Part model, mm, in its own coordinate system. Coordinates: 2 decimals unless noted, no trailing zeros. Write each loop counter-clockwise with the first axis right and the second up, starting at its lowest first coordinate (ties: lowest second). Pieces come first, ordered by that corner, then holes. Notation, with made-up numbers: (-25, 53.5) - (-17, 53.5) arc R5 ccw to (-17, 61.5) - close; hole circle Ø8 at (-27, 67). An arc over 180 degrees is marked (long way). Use a Markdown table: item, result.
```python
from build123d import *

# Parameters (mm, degrees)
SKETCH2_W           = 630
SKETCH2_H           = 6.2
SKETCH2_W_2         = 51.63
SKETCH2_H_2         = 51.63
BOSS_EXTRUDE1_DEPTH = 30
SKETCH2_5_W         = 14
SKETCH2_5_H         = 99
BOSS_EXTRUDE2_DEPTH = 14


with BuildPart() as part:
    # Sketch2 → Boss-Extrude1 (new body)
    # profile 1 of 2: a face of its own
    with BuildSketch(Plane(origin=(0, 0, 0), x_dir=(1, 0, 0), z_dir=(0, 1, 0))):
        Polygon((-320, -34), (-320, -65), (320, -65), (320, -34), (320, 65), (-320, 65), align=None)
        with Locations((0, -51.56)):
            Rectangle(SKETCH2_W, SKETCH2_H, mode=Mode.SUBTRACT)
        with Locations((0, 4.815)):
            Rectangle(SKETCH2_W_2, SKETCH2_H_2, mode=Mode.SUBTRACT)
    # profile 2 of 2: a face of its own
    with BuildSketch(Plane(origin=(0, 0, 0), x_dir=(1, 0, 0), z_dir=(0, 1, 0))):
        with Locations((0, -51.56)):
            Rectangle(SKETCH2_W, SKETCH2_H)
    extrude(amount=BOSS_EXTRUDE1_DEPTH)

    # Sketch2_5 → Boss-Extrude2 (add)
    with BuildSketch(Plane(origin=(0, 0, 0), x_dir=(1, 0, 0), z_dir=(0, 1, 0))):
        with Locations((-327, 15.5)):
            Rectangle(SKETCH2_5_W, SKETCH2_5_H)
        with Locations((327, 15.5)):
            Rectangle(SKETCH2_5_W, SKETCH2_5_H)
    extrude(amount=BOSS_EXTRUDE2_DEPTH)


solid = part.part
```
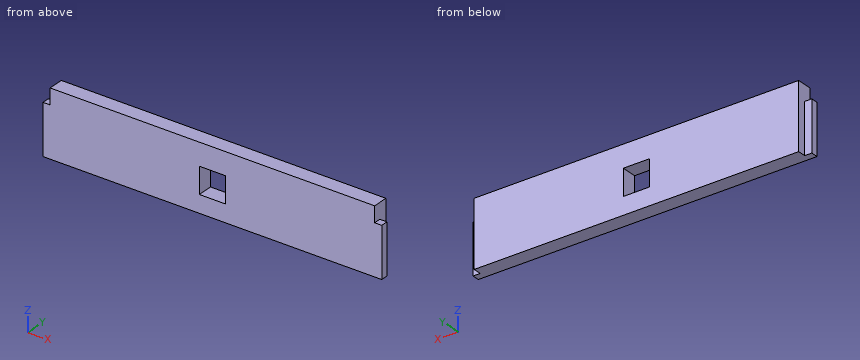
Item 1: Band-saw the part on B-B, the plane y = 4.5. Give the cut face in (x, z) (3 decimals).
From the geometry:
| item | result |
|---|---|
| outline | (-334, -65) - (334, -65) - (334, 34) - (320, 34) - (320, 65) - (-320, 65) - (-320, 34) - (-334, 34) - close; hole (-25.815, -30.63) - (25.815, -30.63) - (25.815, 21) - (-25.815, 21) - close |
Item 2: Drill centre lines: probe 1 along X at (y, z) = (19, 8.5) (3 decimals); probe 2 along Z at (x, y) = (18, 22); probe 3 along X at (y, z) = (13.25, 8) (3 decimals). Where is each one in solid material? Low to high.
From the geometry:
| item | result |
|---|---|
| probe 1 | -320 to -25.815, 25.815 to 320 |
| probe 2 | -65 to -30.63, 21 to 65 |
| probe 3 | -334 to -25.815, 25.815 to 334 |
Item 3: Drop flat-ended pins along their axis: P1, Ø11, axis at x = 327.5, z = -39, coming from the +Y side; P2, Ø7, axis at x = 326, y = 5.5, coming from the +Z side; P3, Ø10, axis at y = 17.5, z = 44, coming from the -X side. Give the stop position or say it passes through.
From the geometry:
| item | result |
|---|---|
| P1 | y = 14 |
| P2 | z = 34 |
| P3 | x = -320 |
Item 4: Band-saw the part on C-C, the plane z = -48.5. Give the cut face in (x, y), then the cut area to 3 significant figures.
From the geometry:
| item | result |
|---|---|
| outline | (-334, 0) - (334, 0) - (334, 14) - (320, 14) - (320, 30) - (-320, 30) - (-320, 14) - (-334, 14) - close |
| area | 19,600 mm^2 |
Item 5: Band-saw the part on A-A, the plane z = 9.5. Give the cut face in (x, y) (3 decimals), then the cut area to 3 significant figures.
From the geometry:
| item | result |
|---|---|
| outline | (-334, 0) - (-25.815, 0) - (-25.815, 30) - (-320, 30) - (-320, 14) - (-334, 14) - close; (25.815, 0) - (334, 0) - (334, 14) - (320, 14) - (320, 30) - (25.815, 30) - close |
| area | 18,000 mm^2 |
